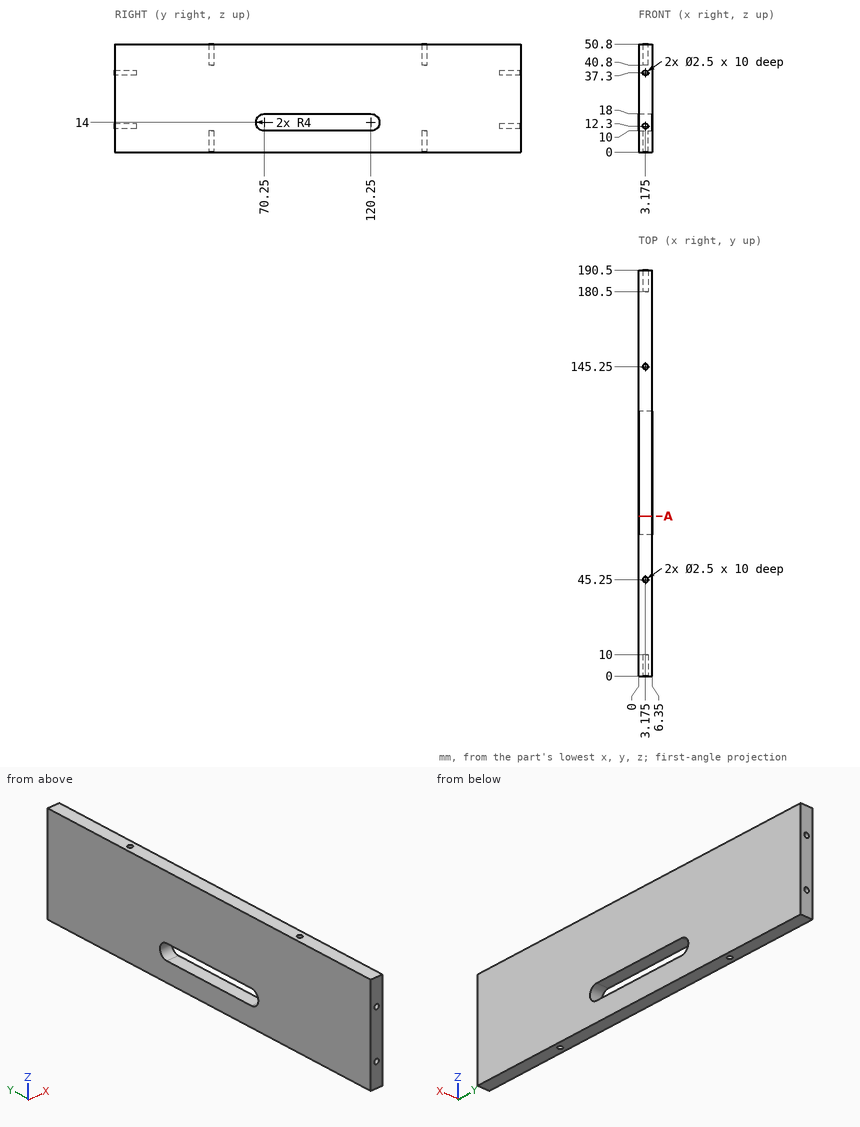
Study the drawing (mm; zero at the part's minimum x, y, z) and answer. Coordinates: 2 decimals unless noted, no trailing zeros. Loops run counter-clockwise (first coordinate to the right, second up) from the corner with the lowest first, then second, coordinate; pieces in that order, holes last. Notation, with made-up numbers: (58, 24.25) -> (86, 24.25) arc R37 cw to (86, 60.25) -> close; hole circle Ø3 at (35.25, -6). An arc over 180 degrees is marked (long way). Write item = value, one per line. Start each with the question number.
1) The part is cut by section A-A, the plane y = 75. Determine the outline of the cut face in (x, z), plus the area to 3 significant figures.
2) Given P1, Ø3, axis at x = 3.175, y = 145.25, coming from the +Z side; P2, Ø1.5, axis at x = 3.175, z = 37.3, coming from the -Y side; P3, Ø1.5, axis at x = 3.175, y = 145.25, coming from the +Z side; P4, Ø2, axis at x = 3.175, y = 45.25, coming from the -Z side, each flat-ended and moving along its own axis, determine where each tip first touches the part or whether it passes through.
3) Find the intervals of material crossed by L1, parallel to Y at x = 3.5, z = 47; L2, parallel to X at y = 145, z = 48; L3, parallel to Y at x = 2.5, z = 14.5, in increasing order. Write a range as from..to.
Result:
q1.outline = (0, 0) -> (6.35, 0) -> (6.35, 10) -> (0, 10) -> close; (0, 18) -> (6.35, 18) -> (6.35, 50.8) -> (0, 50.8) -> close
q1.area = 272 mm²
q2.P1 = 50.8
q2.P2 = 10
q2.P3 = 40.8
q2.P4 = 10
q3.L1 = 0..44.04, 46.46..144.04, 146.46..190.5
q3.L2 = 0..1.95, 4.4..6.35
q3.L3 = 0..66.28, 124.22..190.5
